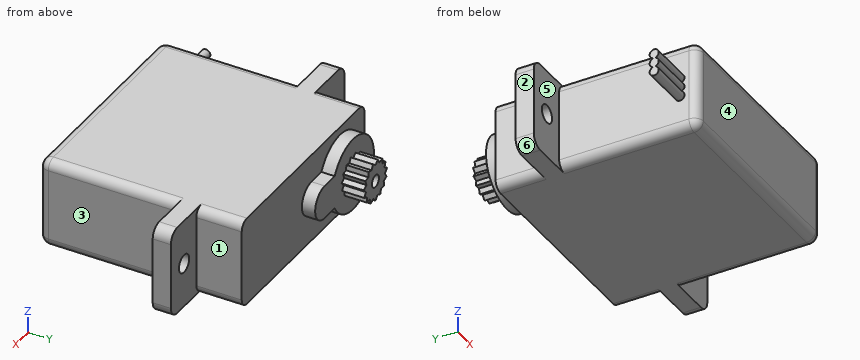
```python
from build123d import *

# Parameters (mm, degrees)
BOSS_EXTRUDE1_DEPTH = 4.925
BOSS_EXTRUDE3_DEPTH = 1.46
SKETCH6_R           = 0.68
BOSS_EXTRUDE4_DEPTH = 2.45
SKETCH2_R           = 0.99
CUT_EXTRUDE6_DEPTH  = 10
FILLET1_R           = 1
FILLET2_R           = 1.25
BOSS_EXTRUDE5_DEPTH = 5


with BuildPart() as part:
    # Sketch1 → Boss-Extrude1 (new body, symmetric)
    with BuildSketch(Plane.XY):
        Polygon((0, 0), (0, 15.3), (-4.925, 15.3), (-4.925, 17.3), (0, 17.3), (0, 22.3), (23.75, 22.3), (23.75, 17.3), (28.675, 17.3), (28.675, 15.3), (23.75, 15.3), (23.75, 0), align=None)
    extrude(amount=BOSS_EXTRUDE1_DEPTH, both=True)

    # Sketch5 → Boss-Extrude3 (add)
    with BuildSketch(Plane(origin=(0, 22.3, 0), x_dir=(1, 0, 0), z_dir=(0, 1, 0))):
        with BuildLine():
            Line((10.25, 1.85), (8.32090644, 1.85))
            ThreePointArc((8.32090644, 1.85), (0.7, 0), (8.32090644, -1.85))
            Line((8.32090644, -1.85), (10.25, -1.85))
            ThreePointArc((10.25, -1.85), (12.1, 0), (10.25, 1.85))
        make_face()
    extrude(amount=BOSS_EXTRUDE3_DEPTH)

    # Sketch6 → Boss-Extrude4 (add)
    with BuildSketch(Plane(origin=(0, 23.76, 0), x_dir=(1, 0, 0), z_dir=(0, 1, 0))):
        Polygon((4.350363372, 1.809573061), (4.735, 2.25), (5.119636628, 1.809573061), (5.650157447, 2.05547728), (5.822402717, 1.49668144), (6.407075857, 1.505543864), (6.337146997, 0.925), (6.874877162, 0.695288237), (6.574865506, 0.193377657), (6.972674265, -0.235189042), (6.494454555, -0.57168144), (6.683557159, -1.125), (6.109817927, -1.237891622), (6.057516818, -1.820288237), (5.48746279, -1.690059097), (5.202801304, -2.200832102), (4.735, -1.85), (4.267198696, -2.200832102), (3.98253721, -1.690059097), (3.412483182, -1.820288237), (3.360182073, -1.237891622), (2.786442841, -1.125), (2.975545445, -0.57168144), (2.497325735, -0.235189042), (2.895134494, 0.193377657), (2.595122838, 0.695288237), (3.132853003, 0.925), (3.062924143, 1.505543864), (3.647597283, 1.49668144), (3.819842553, 2.05547728), align=None)
        with Locations((4.735, 0)):
            Circle(SKETCH6_R, mode=Mode.SUBTRACT)
    extrude(amount=BOSS_EXTRUDE4_DEPTH)

    # Sketch2 → Cut-Extrude6 (cut)
    with BuildSketch(Plane(origin=(0, 17.3, 0), x_dir=(1, 0, 0), z_dir=(0, 1, 0))):
        with Locations((26.125, 0)):
            Circle(SKETCH2_R)
        with Locations((-2.375, 0)):
            Circle(SKETCH2_R)
    extrude(amount=-CUT_EXTRUDE6_DEPTH, mode=Mode.SUBTRACT)

    # Fillet1
    fillet1_edges = [part.edges().sort_by_distance(p)[0] for p in [
        (0, 7.65, -4.925),
        (0, 19.8, -4.925),
        (23.75, 19.8, -4.925),
        (23.75, 7.65, -4.925),
        (11.875, 0, -4.925),
        (23.75, 19.8, 4.925),
        (0, 0, 0),
        (23.75, 0, 0),
        (0, 19.8, 4.925),
        (0, 7.65, 4.925),
        (11.875, 0, 4.925),
        (23.75, 7.65, 4.925),
    ]]
    fillet(fillet1_edges, radius=FILLET1_R)

    # Fillet2
    fillet2_edges = [part.edges().sort_by_distance(p)[0] for p in [
        (-4.925, 16.3, -4.925),
        (28.675, 16.3, 4.925),
        (28.675, 16.3, -4.925),
        (-4.925, 16.3, 4.925),
    ]]
    fillet(fillet2_edges, radius=FILLET2_R)

    # Sketch7 → Boss-Extrude5 (add)
    with BuildSketch(Plane.ZY):
        with BuildLine():
            Line((-0.543660539, 2.20433868), (-0.456339461, 2.20433868))
            ThreePointArc((-0.456339461, 2.20433868), (0, 2.5), (0.456339461, 2.20433868))
            Line((0.456339461, 2.20433868), (0.543660539, 2.20433868))
            ThreePointArc((0.543660539, 2.20433868), (1.5, 2), (0.543660539, 1.79566132))
            Line((0.543660539, 1.79566132), (0.456339461, 1.79566132))
            ThreePointArc((0.456339461, 1.79566132), (0, 1.5), (-0.456339461, 1.79566132))
            Line((-0.456339461, 1.79566132), (-0.543660539, 1.79566132))
            ThreePointArc((-0.543660539, 1.79566132), (-1.5, 2), (-0.543660539, 2.20433868))
        make_face()
    extrude(amount=BOSS_EXTRUDE5_DEPTH)


solid = part.part
```
Source: CAD feature listing. Evaluate the final solid. Frame: model axes, mm. Face numbers are marked on the shaded views. A direction names the side the tool comes from. Round coordinates to 2 decimals unless told otherwise and drop trailing zeros. Loops run counter-clockwise (first coordinate to the right, second up) from the corner with the lowest first, then second, coordinate; pieces in that order, holes last. Notation, with made-up numbers: M -32.5,18 L -1.5,18 A22 ccw -1.5,53 Z; hole C 49,-26.5 d7. An arc over 180 degrees is marked long. Use a Markdown table: item, result. Add a question column.
1. Ray query, line 1 along Y through (x, z) = (22.5, 2.5); line 2 along X through (y, z) = (4.25, 2); line 3 along X through (y, z) = (25.45, 0) (3 decimals). Return the intervals inside material, ascending. Write a range as [from, to].
2. Contact query for flat-ended pins moving along their axis: pin 1 (2.5 mm diameter, centred on x = -2.375, z = 0, fed in from +Y); pin 2 (2.5 mm diameter, centred on y = 9, z = 0.5, fed in from +X); pin 3 (3 mm diameter, centred on x = 12.5, z = 0, fed in from +Y). Output: stop coordinate, or through.
3. Cut plane C-C, the plane z = 3. Output: boundary loops of the cut face in (x, y) (3 decimals), and give its area (3 significant figures).
4. Cut plane B-B, the plane x = 13. Output: boundary loops of the cut face in (y, z) (3 decimals).
5. Set-up query: the marked faces 1, 2 and 3. Return all of +Z, -Z, +X, -X, +Y, -Y with unobstructed straight access to the full face (end or side cutting, diameter ignored); none if empty.
6. Cut plane A-A, the plane y = 21.5. Output: boundary loops of the cut face in (x, z) (3 decimals), and give its area (3 significant figures).
7. Pull-direction query (Y, two-part tool) for the marked faces 4, 5 and 6; classes: +Y half, -Y half, draft (parallel to the pull), parting line (faces both ways), or undercut.
Solution:
| question | item | result |
|---|---|---|
| 1 | line 1 | y = [0, 22.3] |
| 1 | line 2 | x = [0, 23.75] |
| 1 | line 3 | x = [2.716, 4.055], [5.415, 6.754] |
| 2 | pin 1 | stops at y = 17.3 |
| 2 | pin 2 | stops at x = 23.75 |
| 2 | pin 3 | stops at y = 23.76 |
| 3 | outline | M -4.925,15.3 L 0,15.3 L 0,1 A1 ccw 1,0 L 22.75,0 A1 ccw 23.75,1 L 23.75,15.3 L 28.675,15.3 L 28.675,17.3 L 23.75,17.3 L 23.75,22.3 L 7.433,22.3 L 7.433,23.76 L 2.037,23.76 L 2.037,22.3 L 0,22.3 L 0,17.3 L -4.925,17.3 Z |
| 3 | area | 557 mm2 |
| 4 | outline | M 0,-3.925 A1 ccw 1,-4.925 L 22.3,-4.925 L 22.3,4.925 L 1,4.925 A1 ccw 0,3.925 Z |
| 5 | face 1 | +Z, -Z, +X, +Y |
| 5 | face 2 | +Z, -Z, -X, +Y |
| 5 | face 3 | +Z, -Z, +X, -Y |
| 6 | outline | M 0,-3.925 A1 ccw 1,-4.925 L 22.75,-4.925 A1 ccw 23.75,-3.925 L 23.75,3.925 A1 ccw 22.75,4.925 L 1,4.925 A1 ccw 0,3.925 Z |
| 6 | area | 233 mm2 |
| 7 | face 4 | -Y half |
| 7 | face 5 | undercut |
| 7 | face 6 | draft |
